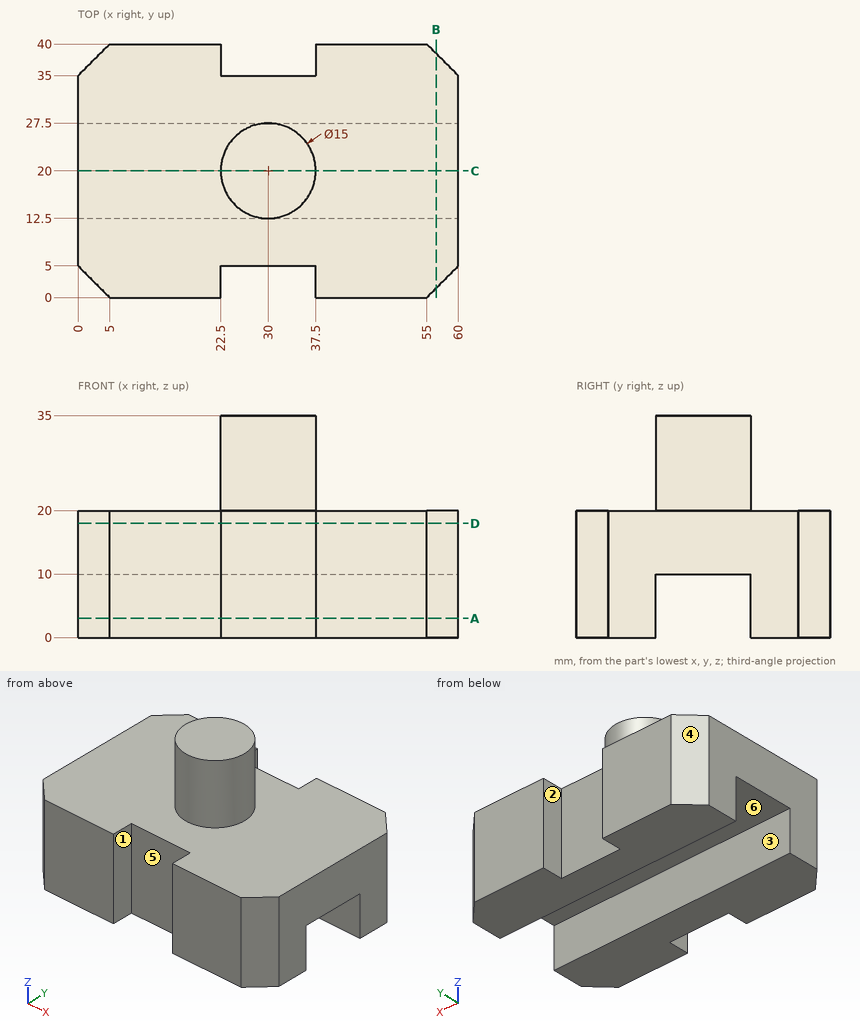
Print and shaded views of the part. All mm, measured from the part's lowest x, y and z. A direction names the side the tool comes from. Round coordinates to 2 decimals unless told otherwise and drop trailing zeros. Loops run counter-clockwise (first coordinate to the right, second up) from the corner with the lowest first, then second, coordinate; pieces in that order, holes last. Notation, with made-up numbers: (-18.75, 77) -> (24.25, 77) arc R27 ccw to (24.25, 104) -> close; hole circle Ø10 at (-34, 63). An arc over 180 degrees is marked (long way). Use CSV: the item, a comma, the result in double quotes. Start each with the question number.
1) Cut at D-D, the plane z = 18. Write the cut outline in (x, y).
2) Cut at A-A, the plane z = 3. Write the cut outline in (x, y).
3) Cut at C-C, the plane y = 20. Write the cut outline in (x, z).
4) Drop flat-ended pins along their axis: P1, Ø1.5, axis at y = 2, z = 6, coming from the +X side; P2, Ø1.5, axis at y = 16, z = 22, coming from the -X side; P3, Ø4.5, axis at x = 30.5, z = 13.5, coming from the +Y side. Give the stop position or say it passes through.
5) Pull direction X, two halves, no side cores. Call the marked faces 4, 5 and 6: +X half, -X half, draft (parallel to the pull), parting line (faces both ways), or undercut.
6) Wall check: L1, parallel to Y at x = 27.5, z = 8; L2, parallel to Y at x = 18, z = 4; L3, parallel to Z at x = 23, y = 19.5. Give the ranges that are in metal, low to high. Write a range as [from, to].
7) Cut at B-B, the plane x = 56.5. Write the cut outline in (y, z), plus the area to 3 significant figures.
8) Which spindle directions (+Z, -Z, +X, -X, +Y, -Y) get a long thin tool onto all of the face, cutting with end or side? Do the marked faces 1, 2 and 3. Say none if no direction does.
Determined:
1,outline,"(0, 5) -> (5, 0) -> (22.5, 0) -> (22.5, 5) -> (37.5, 5) -> (37.5, 0) -> (55, 0) -> (60, 5) -> (60, 35) -> (55, 40) -> (37.5, 40) -> (37.5, 35) -> (22.5, 35) -> (22.5, 40) -> (5, 40) -> (0, 35) -> close"
2,outline,"(0, 5) -> (5, 0) -> (22.5, 0) -> (22.5, 5) -> (37.5, 5) -> (37.5, 0) -> (55, 0) -> (60, 5) -> (60, 12.5) -> (0, 12.5) -> close; (0, 27.5) -> (60, 27.5) -> (60, 35) -> (55, 40) -> (37.5, 40) -> (37.5, 35) -> (22.5, 35) -> (22.5, 40) -> (5, 40) -> (0, 35) -> close"
3,outline,"(0, 10) -> (60, 10) -> (60, 20) -> (37.5, 20) -> (37.5, 35) -> (22.5, 35) -> (22.5, 20) -> (0, 20) -> close"
4,P1,"stops at x = 57.75"
4,P2,"stops at x = 23.24"
4,P3,"stops at y = 35"
5,face 4,"-X half"
5,face 5,"undercut"
5,face 6,"draft"
6,L1,"y = [5, 12.5], [27.5, 35]"
6,L2,"y = [0, 12.5], [27.5, 40]"
6,L3,"z = [10, 35]"
7,outline,"(1.5, 0) -> (12.5, 0) -> (12.5, 10) -> (27.5, 10) -> (27.5, 0) -> (38.5, 0) -> (38.5, 20) -> (1.5, 20) -> close"
7,area,"590 mm2"
8,face 1,"+Z, -Z, -Y"
8,face 2,"+Z, -Z, +Y"
8,face 3,"-Z, +X, -X"
